The model under review builds one solid part; all positions refer to its coordinate system, in mm. A direction names the side the tool comes from. Round coordinates to 2 decimals unless told otherwise and drop trailing zeros. Order: outer loops, then holes, each group sorted by start corner. A loop starts at its lowest first (then second) coordinate and runs counter-clockwise, first axis right, second up.
```python
from build123d import *

# Parameters (mm, degrees)
F1_DEPTH = 63.5
F2_DEPTH = 25.4
F3_DEPTH = 15.875
F4_ANGLE = 180
F5_R     = 5.08


with BuildPart() as f1:
    # F0 (on Front) → F1 (new body, symmetric)
    with BuildSketch(Plane.XZ):
        Polygon((22.225, 9.525), (-41.275, 9.525), (-41.275, -9.525), (41.275, -9.525), (41.275, 9.525), align=None)
    extrude(amount=F1_DEPTH, both=True)

    # F0 (on Front) → F2 (join, symmetric)
    with BuildSketch(Plane.XZ):
        with BuildLine():
            Line((22.225, 27.6352), (22.225, 9.525))
            Line((22.225, 9.525), (41.275, 9.525))
            Line((41.275, 9.525), (41.275, 27.6352))
            ThreePointArc((41.275, 27.6352), (45.738693, 38.411507), (56.515, 42.8752))
            Line((56.515, 42.8752), (60.325, 42.8752))
            Line((60.325, 42.8752), (60.325, 61.9252))
            Line((60.325, 61.9252), (56.515, 61.9252))
            add(Edge.make_bspline(
                [(48.419926, 60.955972), (51.017529, 61.304979), (53.713576, 61.627931), (56.515, 61.9252)],
                knots=[105.444957, 105.444957, 105.444957, 105.444957, 110.944423, 110.944423, 110.944423, 110.944423], degree=3))
            ThreePointArc((48.419926, 60.955972), (29.557773, 48.827463), (22.225, 27.6352))
        make_face()
    extrude(amount=F2_DEPTH, both=True)

    # F0 (on Front) → F3 (join)
    with BuildSketch(Plane.XZ):
        with BuildLine():
            add(Edge.make_bspline(
                [(-41.275, 9.525), (-14.999935, 37.993934), (-1.385662, 54.264229), (48.419926, 60.955972)],
                knots=[0, 0, 0, 0, 105.444957, 105.444957, 105.444957, 105.444957], degree=3))
            Line((-41.275, 9.525), (22.225, 9.525))
            Line((22.225, 9.525), (22.225, 27.6352))
            ThreePointArc((22.225, 27.6352), (29.557773, 48.827463), (48.419926, 60.955972))
        make_face()
    extrude(amount=-F3_DEPTH)

    # F0 (on Front) → F4 (revolve, symmetric)
    with BuildSketch(Plane.XZ) as f4_sk:
        Polygon((61.098028, 66.675), (61.098028, 61.9252), (75.06405, 61.9252), (75.06405, 38.1), (111.125, 38.1), (111.125, 66.675), align=None)
        Polygon((75.06405, 61.9252), (61.098028, 61.9252), (61.098028, 42.8752), (61.098028, 38.1), (75.06405, 38.1), align=None)
    revolve(axis=Axis((60.325, 0, 52.3875), (0, 0, 1)), revolution_arc=F4_ANGLE / 2)
    revolve(f4_sk.sketch, axis=Axis((60.325, 0, 52.3875), (0, 0, -1)), revolution_arc=F4_ANGLE / 2)

    # F5
    f5_edges = [f1.edges().sort_by_distance(p)[0] for p in [
        (41.275, -63.5, 0),
        (-41.275, -63.5, 0),
        (-41.275, 63.5, 0),
        (41.275, 63.5, 0),
    ]]
    fillet(f5_edges, radius=F5_R)


solid = f1.part
```
(1) For faces 1 (the flat face through (80, -1, 38.1)), 2 (the flat face through (4, 15.875, 30)), 3 (the flat face through (58, 0, 61.925)), 4 (the cylindrical face through (29.76, -12.88, 49.08)), list the 3-axis set-ups (+Z, -Z, +X, -X, +Y, -Y) from which the entire face can be reached by the end or side of a thin tool; tool diameter is ignored.
Data:
face 1: -Z, +X, +Y, -Y
face 2: +Z, -X, +Y
face 3: +Z, -X, +Y, -Y
face 4: +Z, -X, -Y
(2) Consider section B-B (y = 38). Write out the cut boundary in (x, z) (3 decimals).
Data:
outline: (-41.275, -9.525) - (41.275, -9.525) - (41.275, 9.525) - (-41.275, 9.525) - close; (60.325, 38.1) - (94.039, 38.1) - (94.039, 66.675) - (60.325, 66.675) - close
(3) To check wall thickness, follow probe 1 along X at (y, z) = (53, 3) (3 decimals); probe 2 along Y at (x, z) = (13, 43) (3 decimals); probe 3 along Z at (x, y) = (102, -25.5) (3 decimals). State the ranges of each line that lie inside material, in increasing order.
Data:
probe 1: x = -41.275 to 41.275
probe 2: y = 0 to 15.875
probe 3: z = 38.1 to 66.675
(4) Insertion check: pin 1 (24 mm diameter, centred on x = -13, y = 40, fed in from +Z) (3 decimals); pin 2 (1 mm diameter, centred on x = 27, z = 28.5, fed in from -Y); pin 3 (1.9 mm diameter, centred on x = 59, y = -6, fed in from -Z). Each pin has a flat end and moves straight along its axis. Give the tip position at first contact, or say it passes through.
Data:
pin 1: stops at z = 9.525
pin 2: stops at y = -25.4
pin 3: stops at z = 42.88
(5) Consider section A-A (z = 0.5). Write out the cut boundary in (x, y) (3 decimals).
Data:
outline: (-41.275, -58.42) arc R5.08 ccw to (-36.195, -63.5) - (36.195, -63.5) arc R5.08 ccw to (41.275, -58.42) - (41.275, 58.42) arc R5.08 ccw to (36.195, 63.5) - (-36.195, 63.5) arc R5.08 ccw to (-41.275, 58.42) - close
(6) Draft analysis for pull direction X (two halves, no side actions). For faces 5 (the flat face through (-1, -1, -9.525)), 6 (the cylindrical face through (45.62, -0.36, 38.29)), 7 (the flat face through (22.225, -13, 19)), 8 (the flat face through (58, 0, 42.875)), state which applies: pulls with the +X half, pulls with the -X half, needs draft (parallel to the pull), parting line crosses it, or undercut.
Data:
face 5: needs draft
face 6: undercut
face 7: pulls with the -X half
face 8: undercut
